Source: CAD feature listing. Evaluate the final solid. Frame: model axes, mm. A direction names the side the tool comes from. Coordinates: 2 decimals unless noted, no trailing zeros. Order: outer loops, then holes, each group sorted by start corner. A loop starts at its lowest first (then second) coordinate and runs counter-clockwise, first axis right, second up. Notation, with made-up numbers: (47.5, -40) -> (78.5, -40) arc R22 cw to (78.5, -19) -> close; hole circle Ø6 at (31, 46). An arc over 180 degrees is marked (long way). Write item = value, one per line. Start each with the question number.
Item 1: Section query C-C (z = 4.5). Output: boundary loops of the cut face in (x, y), then the cut area to 3 significant figures.
Item 2: Set-up query: faces 1 (the flat face through (-14, 15, 7.1)), 2 (the cylindrical face through (18.797, 18.859, 5.574)). Return all of +Z, -Z, +X, -X, +Y, -Y with unobstructed straight access to the full face (end or side cutting, diameter ignored); none if empty.
Item 3: Mould query, pull axis X, two halves, no side actions, for faces 3 (the flat face through (18, 15, 7.1)), 4 (the flat face through (0, 20, 5)), 5 (the flat face through (20, 0, 5)). Classes: released by +X, released by -X, zero draft, split by the parting line, or undercut.
Item 4: Section query D-D (z = 9.5). Output: boundary loops of the cut face in (x, y).
Item 5: Section query A-A (x = 0). Output: boundary loops of the cut face in (y, z).
Item 6: Ray query, line 1 along Y through (x, z) = (16, 2.5); line 2 along Y through (x, z) = (16, 7.9); line 3 along Y through (x, z) = (0.5, 8.75). Return the intervals inside material, ascending. Write a range as [from, to].
```python
from build123d import *

# Parameters (mm, degrees)
SKETCH038_W         = 40
SKETCH038_H         = 40
PAD011_DEPTH        = 11
SKETCH039_R         = 19
POCKET010_DEPTH     = 11.001
HOLE002_D           = 3.9
HOLE002_DEPTH       = 25
HOLE002_CBORE_D     = 6.1
HOLE002_CBORE_DEPTH = 3.9
FILLET012_R         = 4
FILLET014_R         = 0.5
FILLET015_R         = 0.25


with BuildPart() as part:
    # Sketch038 → Pad011 (new body)
    with BuildSketch(Plane.XY):
        Rectangle(SKETCH038_W, SKETCH038_H)
    extrude(amount=PAD011_DEPTH)

    # Sketch039 (on Face6 of Pad011) → Pocket010 (cut, through all)
    with BuildSketch(Plane.XY.offset(11)):
        Circle(SKETCH039_R)
    extrude(amount=-POCKET010_DEPTH, mode=Mode.SUBTRACT)

    # Hole002
    with Locations(Plane.XY.offset(11)):
        with Locations((16, 16), (16, -16), (-16, 16), (-16, -16)):
            CounterBoreHole(HOLE002_D / 2, HOLE002_CBORE_D / 2, HOLE002_CBORE_DEPTH, depth=HOLE002_DEPTH)

    # Fillet012
    fillet012_edges = [part.edges().sort_by_distance(p)[0] for p in [
        (20, 20, 5.5),
        (-20, 20, 5.5),
        (-20, -20, 5.5),
        (20, -20, 5.5),
    ]]
    fillet(fillet012_edges, radius=FILLET012_R)

    # Fillet014
    fillet014_edges = [part.edges().sort_by_distance(p)[0] for p in [
        (-19, 0, 11),
        (19, 0, 5.5),
        (-19, 0, 0),
    ]]
    fillet(fillet014_edges, radius=FILLET014_R)

    # Fillet015
    fillet015_edges = [part.edges().sort_by_distance(p)[0] for p in [
        (0, -20, 0),
        (16, -20, 5.5),
        (-16, -20, 5.5),
        (0, -20, 11),
        (20, 0, 0),
        (20, 16, 5.5),
        (20, -16, 5.5),
        (20, 0, 11),
        (0, 20, 0),
        (-16, 20, 5.5),
        (16, 20, 5.5),
        (0, 20, 11),
        (-20, 0, 0),
        (-20, -16, 5.5),
        (-20, 16, 5.5),
        (-20, 0, 11),
    ]]
    fillet(fillet015_edges, radius=FILLET015_R)


solid = part.part
```
Computed:
q1.outline = (-20, -16) arc R4 ccw to (-16, -20) -> (16, -20) arc R4 ccw to (20, -16) -> (20, 16) arc R4 ccw to (16, 20) -> (-16, 20) arc R4 ccw to (-20, 16) -> close; hole circle Ø38 at (0, 0); hole circle Ø3.9 at (-16, -16); hole circle Ø3.9 at (-16, 16); hole circle Ø3.9 at (16, -16); hole circle Ø3.9 at (16, 16)
q1.area = 404 mm^2
q2.face_1 = +Z
q2.face_2 = +Z, -Z, +X, +Y
q3.face_3 = undercut
q3.face_4 = zero draft
q3.face_5 = released by +X
q4.outline = (-20, -16) arc R4 ccw to (-16, -20) -> (16, -20) arc R4 ccw to (20, -16) -> (20, 16) arc R4 ccw to (16, 20) -> (-16, 20) arc R4 ccw to (-20, 16) -> close; hole circle Ø6.1 at (-16, -16); hole circle Ø6.1 at (-16, 16); hole circle Ø38 at (0, 0); hole circle Ø6.1 at (16, -16); hole circle Ø6.1 at (16, 16)
q5.outline = (-20, 0.25) arc R0.25 ccw to (-19.75, 0) -> (-19.5, 0) arc R0.5 ccw to (-19, 0.5) -> (-19, 10.5) arc R0.5 ccw to (-19.5, 11) -> (-19.75, 11) arc R0.25 ccw to (-20, 10.75) -> close; (19, 0.5) arc R0.5 ccw to (19.5, 0) -> (19.75, 0) arc R0.25 ccw to (20, 0.25) -> (20, 10.75) arc R0.25 ccw to (19.75, 11) -> (19.5, 11) arc R0.5 ccw to (19, 10.5) -> close
q6.line_1 = [-20, -17.95], [-14.05, -10.25], [10.25, 14.05], [17.95, 20]
q6.line_2 = [-20, -19.05], [-12.95, -10.25], [10.25, 12.95], [19.05, 20]
q6.line_3 = [-20, -18.99], [18.99, 20]
